Check sheet for the modelled part. Datum: model origin and axes. Units: mm. A direction names the side the tool comes from. Round coordinates to 2 decimals unless told otherwise and drop trailing zeros. Write each loop counter-clockwise with the first axis right and the second up, starting at its lowest first coordinate (ties: lowest second). Pieces come first, ordered by that corner, then holes. Notation, with made-up numbers: M 7,-1.5 L 13,-1.5 A29 cw 13,29.5 Z; hole C 23.25,55.5 d3. An arc over 180 degrees is marked long. Answer in a Markdown table with one row per item.
```python
from build123d import *

# Parameters (mm, degrees)
BOSS_EXTRUDE1_DEPTH = 76.2
SKETCH3_R           = 12.7
SKETCH3_R_2         = 10
CUT_EXTRUDE1_DEPTH  = 7.35


with BuildPart() as part:
    # Sketch2 → Boss-Extrude1 (new body, symmetric)
    with BuildSketch(Plane.XY):
        with BuildLine():
            Line((-50.8, 0), (50.8, 0))
            Line((50.8, 0), (50.8, 152.4))
            Line((50.8, 152.4), (47.625, 152.4))
            ThreePointArc((47.625, 152.4), (45.37993597, 151.47006403), (44.45, 149.225))
            Line((44.45, 149.225), (44.45, 9.525))
            ThreePointArc((44.45, 9.525), (43.52006403, 7.27993597), (41.275, 6.35))
            Line((41.275, 6.35), (-47.625, 6.35))
            ThreePointArc((-47.625, 6.35), (-49.87006403, 5.42006403), (-50.8, 3.175))
            Line((-50.8, 3.175), (-50.8, 0))
        make_face()
    extrude(amount=BOSS_EXTRUDE1_DEPTH, both=True)

    # Sketch3 → Cut-Extrude1 (cut, through all)
    with BuildSketch(Plane(origin=(0, 6.35, 0), x_dir=(1, 0, 0), z_dir=(0, 1, 0))):
        with Locations((0, 52.5)):
            Circle(SKETCH3_R)
        with Locations((0, -52.5)):
            Circle(SKETCH3_R)
        Circle(SKETCH3_R_2)
    extrude(amount=-CUT_EXTRUDE1_DEPTH, mode=Mode.SUBTRACT)


solid = part.part
```
1. Section check B-B, the plane z = 52.5. Record the cut outline in (x, y) (3 decimals), and give its area (3 significant figures).
Found:
| item | result |
|---|---|
| outline | M -50.8,0 L -12.7,0 L -12.7,6.35 L -47.625,6.35 A3.175 ccw -50.8,3.175 Z; M 12.7,0 L 50.8,0 L 50.8,152.4 L 47.625,152.4 A3.175 ccw 44.45,149.225 L 44.45,9.525 A3.175 cw 41.275,6.35 L 12.7,6.35 Z |
| area | 1,410 mm2 |
2. Section check C-C, the plane z = 0. Record the cut outline in (x, y) (3 decimals), and give its area (3 significant figures).
Found:
| item | result |
|---|---|
| outline | M -50.8,0 L -10,0 L -10,6.35 L -47.625,6.35 A3.175 ccw -50.8,3.175 Z; M 10,0 L 50.8,0 L 50.8,152.4 L 47.625,152.4 A3.175 ccw 44.45,149.225 L 44.45,9.525 A3.175 cw 41.275,6.35 L 10,6.35 Z |
| area | 1,440 mm2 |
3. Scan lines: L1, parallel to Z at x = 0, y = 2.25; L2, parallel to Y at x = 4, z = 70.5; L3, parallel to X at y = 26.5, z = -33.5. Record each from-to range of solid material in increasing order.
Found:
| item | result |
|---|---|
| L1 | z = -76.2 to -65.2, -39.8 to -10, 10 to 39.8, 65.2 to 76.2 |
| L2 | y = 0 to 6.35 |
| L3 | x = 44.45 to 50.8 |
4. Section check D-D, the plane z = 37. Record the cut outline in (x, y) (3 decimals).
Found:
| item | result |
|---|---|
| outline | M -50.8,0 L 50.8,0 L 50.8,152.4 L 47.625,152.4 A3.175 ccw 44.45,149.225 L 44.45,9.525 A3.175 cw 41.275,6.35 L -47.625,6.35 A3.175 ccw -50.8,3.175 Z |
5. Go/stop test with flat-tipped pins: pin 1 (2 mm diameter, centred on x = 2.5, z = 23.5, fed in from -Y); pin 2 (2 mm diameter, centred on y = 56.5, z = -30.5, fed in from -X). Record where each tip stops, or that it passes through.
Found:
| item | result |
|---|---|
| pin 1 | stops at y = 0 |
| pin 2 | stops at x = 44.45 |
6. Section check A-A, the plane x = 0. Record the cut outline in (y, z).
Found:
| item | result |
|---|---|
| outline | M 0,-76.2 L 6.35,-76.2 L 6.35,-65.2 L 0,-65.2 Z; M 0,-39.8 L 6.35,-39.8 L 6.35,-10 L 0,-10 Z; M 0,10 L 6.35,10 L 6.35,39.8 L 0,39.8 Z; M 0,65.2 L 6.35,65.2 L 6.35,76.2 L 0,76.2 Z |
7. Draft check along X on faces 3 (the face through (45, 54, -76.2)), 4 (the face through (-2.17, 3.22, 9.76)), 5 (the face through (50.8, 75, 1)). Enter one of: +X half, -X half, draft (parallel to the pull), parting line (faces both ways), or undercut.
Found:
| item | result |
|---|---|
| face 3 | draft |
| face 4 | undercut |
| face 5 | +X half |
8. Access from +Z, -Z, +X, -X, +Y, -Y to the whole of each face (thin tool, end or side, straight path). Record for faces 1 (the face through (44.45, 80, 1)), 2 (the face through (-1.653, 3.219, -65.092)).
Found:
| item | result |
|---|---|
| face 1 | +Z, -Z, -X, +Y |
| face 2 | +Y, -Y |
